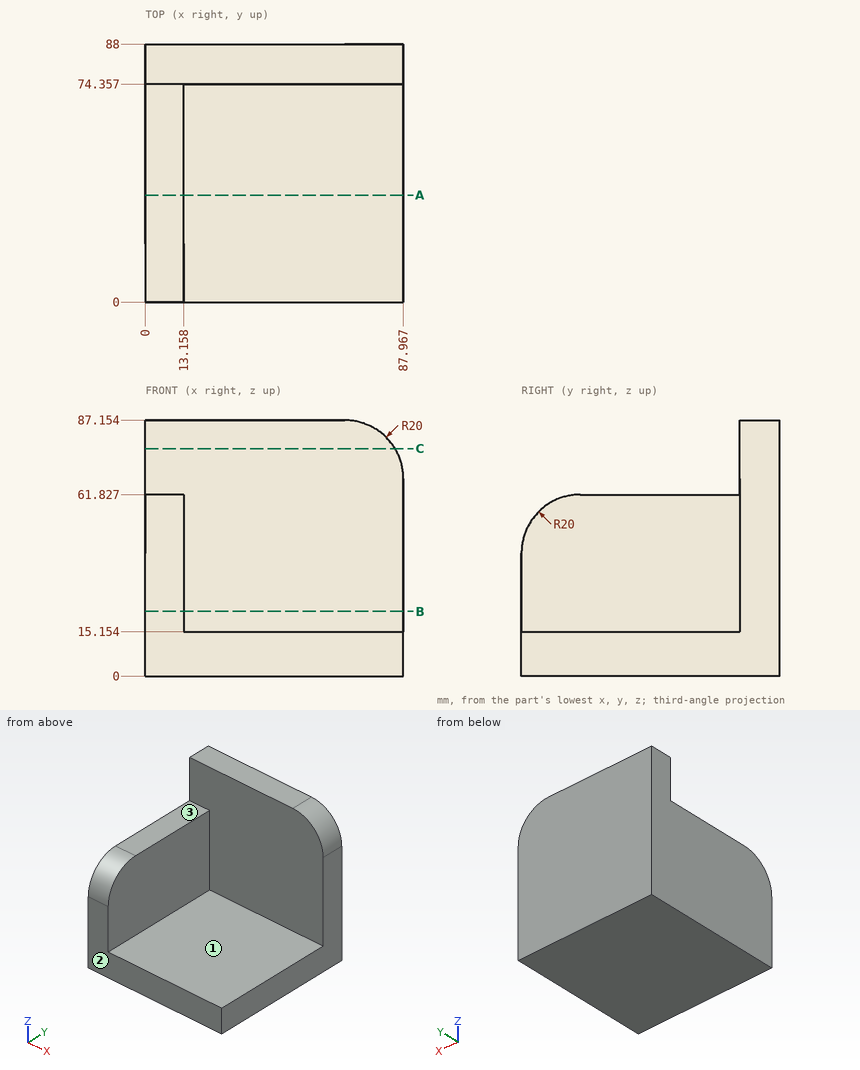
Could you check a few things on this drawing? It's one solid part, dimensions in mm from its lowest x, y, z. A direction names the side the tool comes from. Coordinates: 2 decimals unless noted, no trailing zeros. Write each loop counter-clockwise with the first axis right and the second up, starting at its lowest first coordinate (ties: lowest second). Pieces come first, ordered by that corner, then holes.
1) Which directions (+Z, -Z, +X, -X, +Y, -Y) give clear straight access to the entire face, cutting with the end or side of a thin tool? Please do the marked faces 1, 2 and 3.
Filled in:
face 1: +Z, +X, -Y
face 2: +Z, -Z, +X, -X, -Y
face 3: +Z, +X, -X, -Y
2) If we section it at C-C (z = 77.5): List the corners of the cut face in (x, y) for me, plus the area to 3 significant figures.
Filled in:
outline: (0, 74.36) - (85.08, 74.36) - (85.08, 88) - (0, 88) - close
area: 1,160 mm2
3) If we section it at A-A (y = 36.5): List the corners of the cut face in (x, z) for me.
Filled in:
outline: (0, 0) - (87.97, 0) - (87.97, 15.15) - (13.16, 15.15) - (13.16, 61.83) - (0, 61.83) - close
4) If I drill on line 1 (X direction, y = 15, z = 49); line 2 (Y direction, x = 38, z = 45); line 3 (Z direction, x = 28, y = 17.5), over which ranges is the centre line in solid material (lowest first)?
Filled in:
line 1: x = 0 to 13.16
line 2: y = 74.36 to 88
line 3: z = 0 to 15.15
5) I'm going to push flat-ended pins straight in: pin 1 (12 mm diameter, centred on x = 18.5, z = 50.5, fed in from -Y); pin 2 (3 mm diameter, centred on y = 27, z = 19, fed in from +X); pin 3 (4 mm diameter, centred on x = 6.5, y = 54.5, fed in from +Z). Where does each tip first touch, or does it pass through?
Filled in:
pin 1: stops at y = 0.9
pin 2: stops at x = 13.16
pin 3: stops at z = 61.83
6) If we section it at B-B (z = 22): List the corners of the cut face in (x, y) for me.
Filled in:
outline: (0, 0) - (13.16, 0) - (13.16, 74.36) - (87.97, 74.36) - (87.97, 88) - (0, 88) - close
